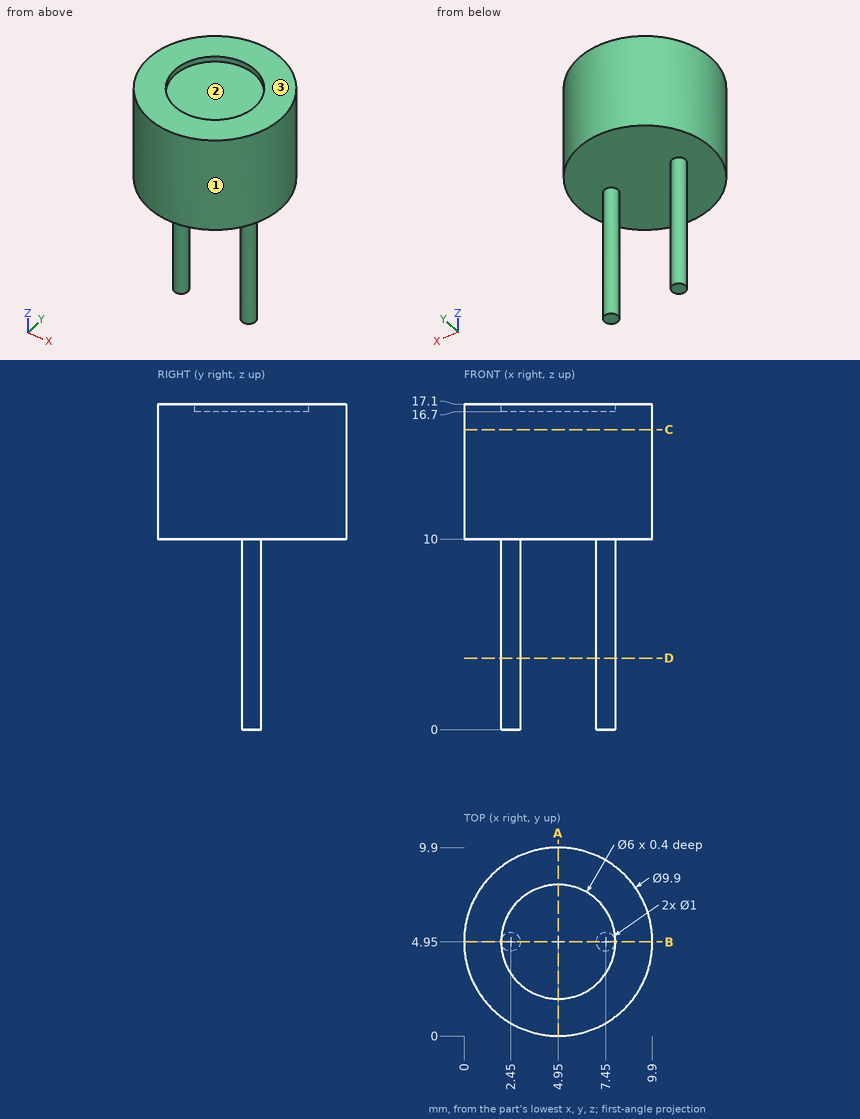
Verification items for this drawing (mm, ordinates from the low corner). Coordinates: 2 decimals unless noted, no trailing zeros. Order: outer loops, then holes, each group sorted by start corner. A loop starts at its lowest first (then second) coordinate and runs counter-clockwise, first axis right, second up. Notation, with made-up numbers: M 43.5,-34.5 L 96.5,-34.5 A22 cw 96.5,-2.5 Z; hole C 4,25 d6. An arc over 180 degrees is marked long. One line per item, written item: value. Start each with the question number.
Item 1: Thickness scan on probe 1 along Z at (x, y) = (1.5, 4); probe 2 along Y at (x, z) = (4.95, 16.9); probe 3 along Z at (x, y) = (4.5, 6.75). Record the ranges inside material, lowest first.
Item 2: Sectioned sample at D-D on z = 3.75. Record the cut outline in (x, y).
Item 3: Sectioned sample at B-B on y = 4.95. Record the cut outline in (x, z), then the cut area to 3 significant figures.
Item 4: Mould release check, pull along X, two halves, no side actions. Record for the marked faces 1, 2 and 3: pulls with the +X half, pulls with the -X half, needs draft (parallel to the pull), parting line crosses it, or undercut.
Item 5: Depth check by flat-ended pin: P1, Ø1, axis at y = 8.5, z = 14.5, coming from the -X side; P2, Ø1, axis at x = 9, z = 10, coming from the -Y side; P3, Ø4, axis at y = 6.5, z = 5.5, coming from the +X side. Enter the tip coordinate at first touch or a pass-through.
Item 6: Sectioned sample at A-A on x = 4.95. Record the cut outline in (y, z).
Item 7: Sectioned sample at C-C on z = 15.75. Record the cut outline in (x, y).
Calculated:
1. probe 1: 10 to 17.1
1. probe 2: 0 to 1.95, 7.95 to 9.9
1. probe 3: 10 to 16.7
2. outline: C 2.45,4.95 d1; C 7.45,4.95 d1
3. outline: M 0,10 L 1.95,10 L 1.95,0 L 2.95,0 L 2.95,10 L 6.95,10 L 6.95,0 L 7.95,0 L 7.95,10 L 9.9,10 L 9.9,17.1 L 7.95,17.1 L 7.95,16.7 L 1.95,16.7 L 1.95,17.1 L 0,17.1 Z
3. area: 87.9 mm^2
4. face 1: parting line crosses it
4. face 2: undercut
4. face 3: needs draft
5. P1: x = 1.05
5. P2: y = 1.5
5. P3: x = 7.95
6. outline: M 0,10 L 9.9,10 L 9.9,17.1 L 7.95,17.1 L 7.95,16.7 L 1.95,16.7 L 1.95,17.1 L 0,17.1 Z
7. outline: C 4.95,4.95 d9.9
